Autodesk Inventor part; units mm, degrees
ref_plane "YZ Plane" through (0, 0, 0) normal (1, 0, 0) x (0, 1, 0)
ref_plane "XZ Plane" through (0, 0, 0) normal (0, 1, 0) x (-1, 0, 0)
ref_plane "XY Plane" through (0, 0, 0) normal (0, 0, 1) x (1, 0, 0)
sketch "Skizze1" plane through (0, 0, 0) normal (0, 1, 0) x (-1, 0, 0)
  line L0 (-16.35, 12.5) -> (16.35, 12.5)
  line L1 (16.35, 12.5) -> (16.35, -12.5)
  line L2 (16.35, -12.5) -> (-16.35, -12.5)
  line L3 (-16.35, -12.5) -> (-16.35, 12.5)
  line L4 (-16.35, 12.5) -> (16.35, -12.5) construction
  line L5 (16.35, 12.5) -> (-16.35, -12.5) construction
  point P0 (0, 0)
  dimension "d0" = 32.7
  dimension "d1" = 25
extrude "Extrusion1" add sketch "Skizze1" along normal blind 10
sketch "Skizze3" plane through (0, 10, 0) normal (0, 1, 0) x (1, 0, 0)
  line L0 (0, 17.5) -> (0, -17.5)
  line L1 (-16.35, -12.5) -> (16.35, -12.5)
  line L2 (-1.15, -12.5) -> (1.15, -12.5)
  line L3 (1.15, -12.5) -> (1.15, 0.5)
  line L4 (1.15, 0.5) -> (-1.15, 0.5)
  line L5 (-1.15, 0.5) -> (-1.15, -12.5)
  point P0 (0, 0)
  point P1 (1.15, -12.5)
  dimension "d11" = 2.3
  dimension "d12" = 13
extrude "Extrusion2" cut sketch "Skizze3" against normal blind 9
sketch "Skizze4" plane through (0, 10, 0) normal (0, 1, 0) x (1, 0, 0)
  line L0 (-1.15, -12.5) -> (-1.15, 0.5)
  circle A0 centre (0, 4.8506) radius 4.5
  line L1 (0, 17.5) -> (0, -17.5)
  circle A1 centre (0, 4.8506) radius 6
  point P0 (0, 0)
  point P1 (-1.15, -1.0382)
  point P2 (0, 0.3506)
  point P3 (0, 10.8506)
  point P4 (0, 9.3506)
  point P5 (0, -1.1494)
  dimension "d16" = 9
  dimension "d17" = 1.5
extrude "Extrusion3" cut sketch "Skizze4" against normal up to surface (9 mm away) contours A1 L1 A0 L0 | L0 A0 L1 A1 | A1 L1 A0
fillet "Rundung1" radius 3 2 edges at (-1.15, 5.5, 1.0382) (1.15, 5.5, 1.0382)
sketch "Skizze5" plane through (0, 10, 0) normal (0, 1, 0) x (1, 0, 0)
  line L0 (0, 17.5) -> (0, -17.5)
  line L1 (16.35, 12.5) -> (-16.35, 12.5)
  point P0 (0, 0)
  point P1 (-10, 2.5)
  point P2 (10, 2.5)
  dimension "d21" = 10
  dimension "d22" = 20
hole "Bohrung2" at (-10, 10, -2.5) at (10, 10, -2.5) direction (0, -1, 0) diameter 3.4 end through all counterbore diameter 6.5 counterbore depth 3.4
fillet "Rundung2" radius 2 4 edges at (16.35, 5, 12.5) (16.35, 5, -12.5) (-16.35, 5, -12.5) (-16.35, 5, 12.5)
properties part number "19_Belt_holder" material "PET-Kunststoff"
Input: part model. Units: mm. Frame: model coordinates. A direction names the side the tool comes from. Give positions to 0.01 mm unless a question says otherwise; leave off trailing zeros. Loops run counter-clockwise (first coordinate to the right, second up) from the corner with the lowest first, then second, coordinate; pieces in that order, holes last. Notation, with made-up numbers: (56.5, -18) - (96.5, -18) arc R24 cw to (96.5, -8) - close; hole circle Ø7 at (-28, 50.5). An arc over 180 degrees is marked (long way). Use CSV: the item, a comma, the result in double quotes. Start each with the question number.
Item 1: Line query: line 1 (X direction, y = 4.25, z = 6.5); line 2 (Z direction, x = 10, y = 8.85); line 3 (Z direction, x = 4, y = 4.5). Output: solid intervals per line, ascending.
Item 2: Reachability of faces 1 (the flat face through (-1.15, 6, 8)), 2 (the flat face through (3, 5, 12.5)), 3 (the flat face through (11.4, 6.6, -1.1)) from +Z, -Z, +X, -X, +Y, -Y: full face, straight path, thin tool, end or side. Return the list, or none.
Item 3: Section A-A on y = 2.5. Return loops of the section in (x, z), then the cut area to 3 significant figures.
Item 4: Section C-C on z = -2.5. Return loops of the section in (x, y).
Item 5: Section B-B on x = -10. Return loops of the section in (y, z).
Item 6: Section D-D on y = 7.25. Return loops of the section in (x, z), then the cut area to 3 significant figures.
Item 7: Contact query for flat-ended pins moving along their axis: P1, Ø1.1, axis at x = -0.5, y = 7, coming from the +Z side; P2, Ø6, axis at x = -10, z = -2.5, coming from the +Y side; P3, Ø3, axis at x = 10, z = -2.5, coming from the +Y side. Output: stop coordinate, or through.
Item 8: Mould query, pull axis X, two halves, no side actions, for faces 4 (the cylindrical face through (0.224, 5.563, -10.846)), 5 (the flat face through (0, 5, -12.5)), 6 (the flat face through (-16.35, 5, 0)), 7 (the flat face through (0, 1, 0)). Classes: pulls with the +X half, pulls with the -X half, needs draft (parallel to the pull), parting line crosses it, or undercut.
Ans:
1,line 1,"x = -16.35 to -1.15, 1.15 to 16.35"
1,line 2,"z = -12.5 to -5.75, 0.75 to 12.5"
1,line 3,"z = -12.5 to -9.32, -6.91 to -2.79, -0.38 to 12.5"
2,face 1,"+Z, +Y"
2,face 2,"+Z, +X, -X, +Y, -Y"
2,face 3,"+Y"
3,outline,"(-16.35, -10.5) arc R2 ccw to (-14.35, -12.5) - (14.35, -12.5) arc R2 ccw to (16.35, -10.5) - (16.35, 10.5) arc R2 ccw to (14.35, 12.5) - (1.15, 12.5) - (1.15, 3.14) arc R3 ccw to (2.77, 0.47) arc R6 cw (long way) to (-2.77, 0.47) arc R3 ccw to (-1.15, 3.14) - (-1.15, 12.5) - (-14.35, 12.5) arc R2 ccw to (-16.35, 10.5) - close; (-1.15, -0.5) arc R4.5 ccw (long way) to (1.15, -0.5) - close; hole circle Ø3.4 at (-10, -2.5); hole circle Ø3.4 at (10, -2.5)"
3,area,"719 mm2"
4,outline,"(-16.35, 0) - (-11.7, 0) - (-11.7, 6.6) - (-13.25, 6.6) - (-13.25, 10) - (-16.35, 10) - close; (-8.3, 0) - (8.3, 0) - (8.3, 6.6) - (6.75, 6.6) - (6.75, 10) - (5.52, 10) - (5.52, 1) - (3.84, 1) - (3.84, 10) - (-3.84, 10) - (-3.84, 1) - (-5.52, 1) - (-5.52, 10) - (-6.75, 10) - (-6.75, 6.6) - (-8.3, 6.6) - close; (11.7, 0) - (16.35, 0) - (16.35, 10) - (13.25, 10) - (13.25, 6.6) - (11.7, 6.6) - close"
5,outline,"(0, -12.5) - (10, -12.5) - (10, -5.75) - (6.6, -5.75) - (6.6, -4.2) - (0, -4.2) - close; (0, -0.8) - (6.6, -0.8) - (6.6, 0.75) - (10, 0.75) - (10, 12.5) - (0, 12.5) - close"
6,outline,"(-16.35, -10.5) arc R2 ccw to (-14.35, -12.5) - (14.35, -12.5) arc R2 ccw to (16.35, -10.5) - (16.35, 10.5) arc R2 ccw to (14.35, 12.5) - (1.15, 12.5) - (1.15, 3.14) arc R3 ccw to (2.77, 0.47) arc R6 cw (long way) to (-2.77, 0.47) arc R3 ccw to (-1.15, 3.14) - (-1.15, 12.5) - (-14.35, 12.5) arc R2 ccw to (-16.35, 10.5) - close; (-1.15, -0.5) arc R4.5 ccw (long way) to (1.15, -0.5) - close; hole circle Ø6.5 at (-10, -2.5); hole circle Ø6.5 at (10, -2.5)"
6,area,"670 mm2"
7,P1,"stops at z = -0.5"
7,P2,"stops at y = 6.6"
7,P3,"passes through"
8,face 4,"undercut"
8,face 5,"needs draft"
8,face 6,"pulls with the -X half"
8,face 7,"undercut"
